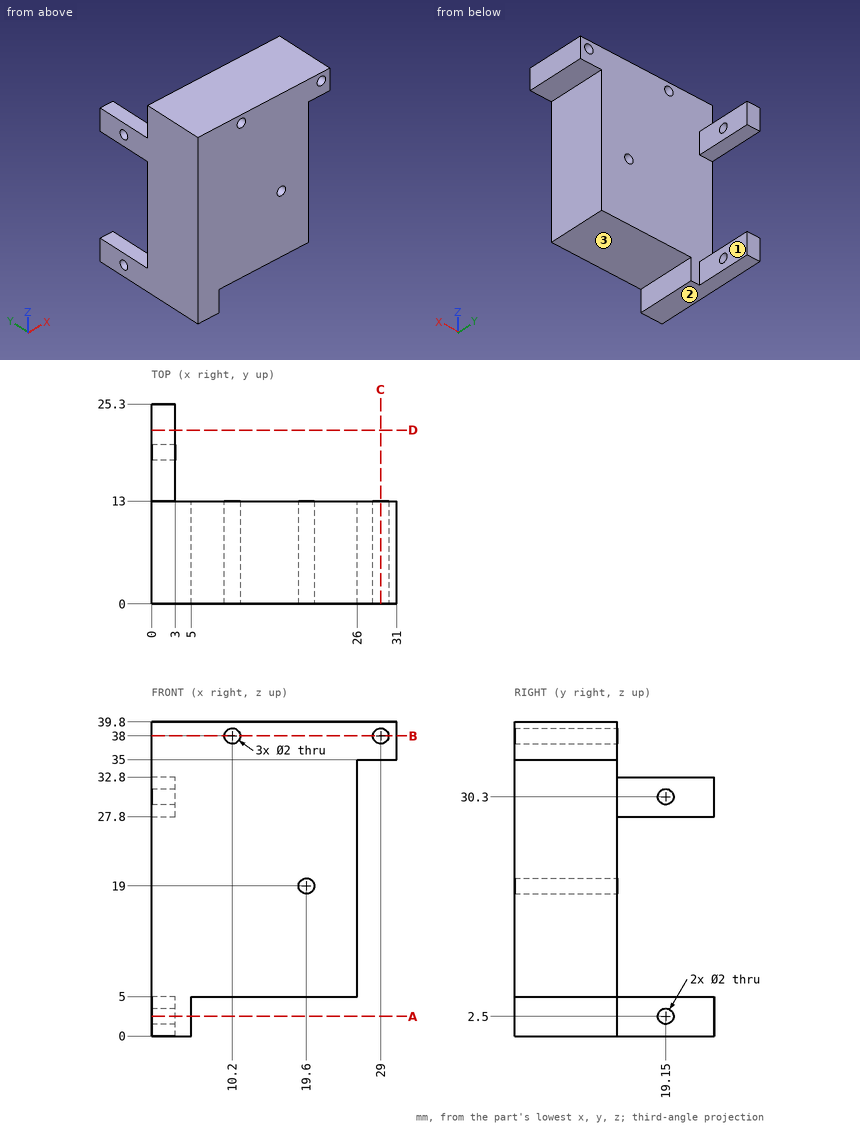
Geometry: see drawing. Coordinates: mm, zero at the bounding-box minimum. A direction names the side the tool comes from. Coordinates: 2 decimals unless noted, no trailing zeros. Loops run counter-clockwise (first coordinate to the right, second up) from the corner with the lowest first, then second, coordinate; pieces in that order, holes last. Notation, with made-up numbers: (67.25, 55.25) - (117.25, 55.25) arc R26 cw to (117.25, 74.25) - close; hole circle Ø5 at (21.5, 43). An arc over 180 degrees is marked (long way). Return JSON: item names as keys, results as strings.
Q1. Section A-A, the plane z = 2.5. Return loops of the section in (x, y), plus the area to 3 significant figures.
Results:
{"outline": "(0, 0) - (5, 0) - (5, 13) - (3, 13) - (3, 18.15) - (0, 18.15) - close; (0, 20.15) - (3, 20.15) - (3, 25.3) - (0, 25.3) - close", "area": "95.9 mm2"}
Q2. Section C-C, the plane x = 29. Return loops of the section in (y, z).
Results:
{"outline": "(0, 35) - (13, 35) - (13, 37) - (0, 37) - close; (0, 39) - (13, 39) - (13, 39.8) - (0, 39.8) - close"}
Q3. Section B-B, the plane z = 38. Return loops of the section in (x, y), plus the area to 3 significant figures.
Results:
{"outline": "(0, 0) - (9.2, 0) - (9.2, 13) - (0, 13) - close; (11.2, 0) - (28, 0) - (28, 13) - (11.2, 13) - close; (30, 0) - (31, 0) - (31, 13) - (30, 13) - close", "area": "351 mm2"}
Q4. Access query for the marked faces 1, 2 and 3. Directions: +Z, -Z, +X, -X, +Y, -Y. A direction counts if a zero-diameter tool reaches every point of the face in a straight line with its end or side. Return the directions, or none.
Results:
{"face 1": "+Z, -Z, +X, +Y", "face 2": "-Z, +X, -X, +Y, -Y", "face 3": "-Z, +X, +Y, -Y"}
Q5. Contact query for flat-ended pins moving along their axis: P1, Ø2.5, axis at x = 2, y = 20, coming from the +Z side; P2, Ø1.6, axis at y = 19.15, z = 30.3, coming from the -X side; P3, Ø8, axis at x = 16, z = 10, coming from the -Y side; P4, Ø2, axis at y = 12, z = 8.5, coming from the +X side. Output: stop coordinate, or through.
Results:
{"P1": "z = 32.8", "P2": "through", "P3": "y = 0", "P4": "x = 26"}
Q6. Section D-D, the plane y = 22. Return loops of the section in (x, z), plus the area to 3 significant figures.
Results:
{"outline": "(0, 0) - (3, 0) - (3, 5) - (0, 5) - close; (0, 27.8) - (3, 27.8) - (3, 32.8) - (0, 32.8) - close", "area": "30.0 mm2"}
Q7. Material intervals for line 1 along X through (y, z) = (4.5, 38); line 2 along Y through (x, z) = (2.25, 2.5); line 3 along Z through (x, y) = (19.6, 10.25), sorted ascending.
Results:
{"line 1": "0 to 9.2, 11.2 to 28, 30 to 31", "line 2": "0 to 18.15, 20.15 to 25.3", "line 3": "5 to 18, 20 to 39.8"}
